Drawing for the job (mm, zero at the part's lowest x, y, z). Coordinates: 2 decimals unless noted, no trailing zeros. Loops run counter-clockwise (first coordinate to the right, second up) from the corner with the lowest first, then second, coordinate; pieces in that order, holes last.
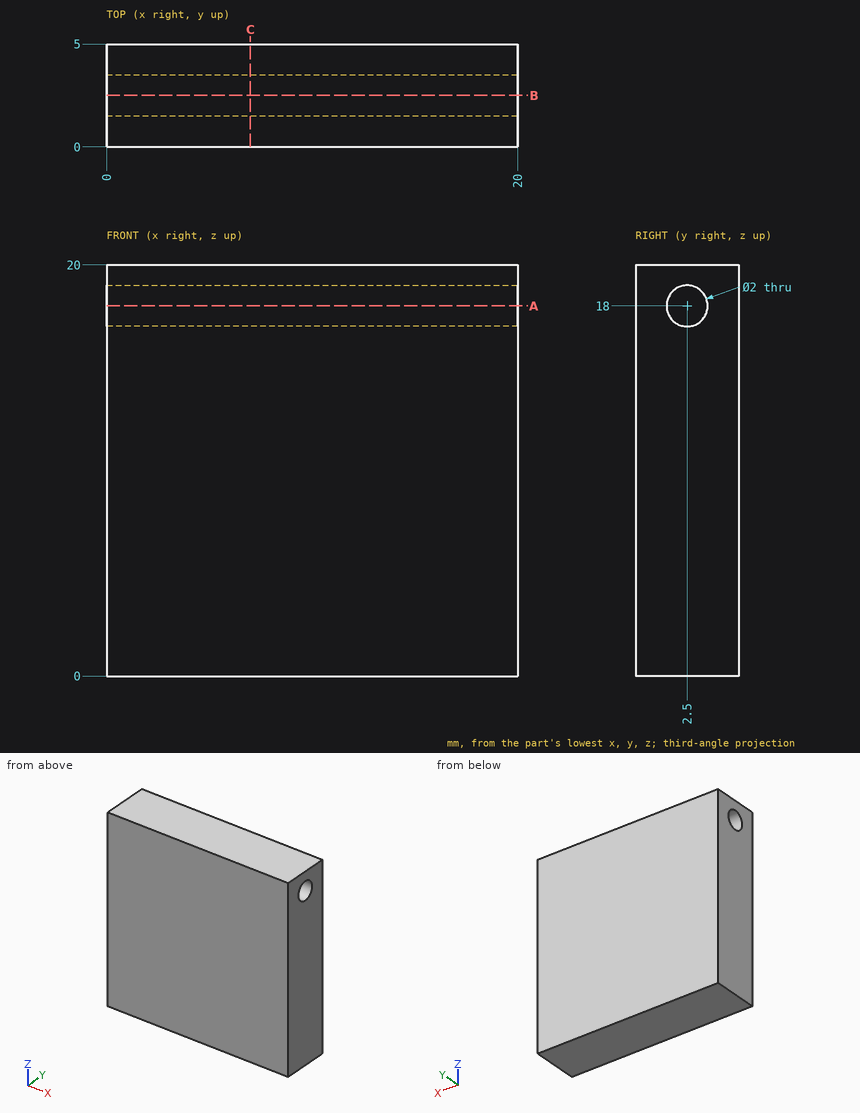
Q1. Saw through at A-A (z = 18). List the corners of the cut face in (x, y), plus the area to 3 significant figures.
Q2. Saw through at B-B (y = 2.5). List the corners of the cut face in (x, z).
Q3. Probe line 1 (Y direction, x = 13.5, z = 18); line 2 (Z direction, x = 5, y = 1.6); line 3 (Z direction, x = 15.5, y = 2.1). List the from-to ranges inside material, lowest first.
Q4. Drop a flat-ended pin along its axis: P1, Ø1.8, axis at y = 2.5, z = 18, coming from the +X side. Give the stop position or say it passes through.
Q5. Saw through at C-C (x = 7). List the corners of the cut face in (y, z), plus the area to 3 significant figures.
Checked values:
1. outline: (0, 0) - (20, 0) - (20, 1.5) - (0, 1.5) - close; (0, 3.5) - (20, 3.5) - (20, 5) - (0, 5) - close
1. area: 60.0 mm2
2. outline: (0, 0) - (20, 0) - (20, 17) - (0, 17) - close; (0, 19) - (20, 19) - (20, 20) - (0, 20) - close
3. line 1: y = 0 to 1.5, 3.5 to 5
3. line 2: z = 0 to 17.56, 18.44 to 20
3. line 3: z = 0 to 17.08, 18.92 to 20
4. P1: passes through
5. outline: (0, 0) - (5, 0) - (5, 20) - (0, 20) - close; hole circle Ø2 at (2.5, 18)
5. area: 96.9 mm2
